Source: CAD feature listing. Evaluate the final solid. Frame: model axes, mm. A direction names the side the tool comes from. Give positions to 0.01 mm unless a question says otherwise; leave off trailing zeros. Loops run counter-clockwise (first coordinate to the right, second up) from the corner with the lowest first, then second, coordinate; pieces in that order, holes last. Notation, with made-up numbers: M 38,-23 L 71,-23 A15 ccw 71,2 Z; hole C 10.5,28 d3. An arc over 180 degrees is marked long. Put each result on its own line as item: value.
from build123d import *

# Parameters (mm, degrees)
F0_W     = 15.4686
F0_H     = 127
F1_DEPTH = 12.7
F2_R     = 2.0193
F3_DEPTH = 6.35
F4_R     = 3.175
F5_DEPTH = 15.875
F6_SIZE  = 1.6002
F8_DEPTH = 25.4


with BuildPart() as f1:
    # F0 (on Right) → F1 (new body)
    with BuildSketch(Plane.YZ):
        Rectangle(F0_W, F0_H)
    extrude(amount=F1_DEPTH)

    # F2 (on Right) → F3 (cut)
    with BuildSketch(Plane.YZ):
        with Locations((0, -55.5625)):
            Circle(F2_R)
    extrude(amount=F3_DEPTH, mode=Mode.SUBTRACT)

    # F4 (on face) → F5 (cut)
    with BuildSketch(Plane(origin=(0, 0, -63.5), x_dir=(1, 0, 0), z_dir=(0, 0, -1))):
        with Locations((6.35, 0)):
            Circle(F4_R)
    extrude(amount=-F5_DEPTH, mode=Mode.SUBTRACT)

    # F6
    f6_edges = [f1.edges().sort_by_distance(p)[0] for p in [
        (6.35, 7.7343, 63.5),
        (6.35, -7.7343, 63.5),
        (0, 0, 63.5),
        (12.7, 0, 63.5),
    ]]
    chamfer(f6_edges, length=F6_SIZE)

    # F7 (on face) → F8 (cut)
    with BuildSketch(Plane(origin=(0, 0, 0), x_dir=(0, -1, 0), z_dir=(-1, 0, 0))):
        Polygon((-3.8227, -43.026294), (-3.8227, -41.502294), (-7.7343, -40.078588), (-7.7343, -44.45), align=None)
        Polygon((-7.7343, 54.206212), (-7.7343, 49.8348), (-3.8227, 51.258506), (-3.8227, 52.782506), align=None)
        Polygon((-7.7343, 48.313412), (-7.7343, 43.942), (-3.8227, 45.365706), (-3.8227, 46.889706), align=None)
        Polygon((-7.7343, 42.420612), (-7.7343, 38.0492), (-3.8227, 39.472906), (-3.8227, 40.996906), align=None)
        Polygon((-7.7343, 36.527812), (-7.7343, 32.1564), (-3.8227, 33.580106), (-3.8227, 35.104106), align=None)
        Polygon((-7.7343, 30.635012), (-7.7343, 26.2636), (-3.8227, 27.687306), (-3.8227, 29.211306), align=None)
        Polygon((-7.7343, 24.742212), (-7.7343, 20.3708), (-3.8227, 21.794506), (-3.8227, 23.318506), align=None)
        Polygon((-7.7343, 18.849412), (-7.7343, 14.478), (-3.8227, 15.901706), (-3.8227, 17.425706), align=None)
        Polygon((-7.7343, 12.956612), (-7.7343, 8.5852), (-3.8227, 10.008906), (-3.8227, 11.532906), align=None)
        Polygon((-7.7343, 7.063812), (-7.7343, 2.6924), (-3.8227, 4.116106), (-3.8227, 5.640106), align=None)
        Polygon((-7.7343, 1.171012), (-7.7343, -3.2004), (-3.8227, -1.776694), (-3.8227, -0.252694), align=None)
        Polygon((-7.7343, -4.721788), (-7.7343, -9.0932), (-3.8227, -7.669494), (-3.8227, -6.145494), align=None)
        Polygon((-7.7343, -10.614588), (-7.7343, -14.986), (-3.8227, -13.562294), (-3.8227, -12.038294), align=None)
        Polygon((-7.7343, -16.507388), (-7.7343, -20.8788), (-3.8227, -19.455094), (-3.8227, -17.931094), align=None)
        Polygon((-7.7343, -22.400188), (-7.7343, -26.7716), (-3.8227, -25.347894), (-3.8227, -23.823894), align=None)
        Polygon((-7.7343, -28.292988), (-7.7343, -32.6644), (-3.8227, -31.240694), (-3.8227, -29.716694), align=None)
        Polygon((-7.7343, -34.185788), (-7.7343, -38.5572), (-3.8227, -37.133494), (-3.8227, -35.609494), align=None)
    extrude(amount=-F8_DEPTH, mode=Mode.SUBTRACT)


solid = f1.part
1. Contact query for a flat-ended pin moving along its axis: P1, Ø0.8, axis at x = 8, z = 22.5, coming from the +Y side. Output: stop coordinate, or through.
Found:
P1: y = 3.82
2. Access query for faces 4 (the flat face through (6, 7.734, -54)), 5 (the flat face through (6.261, 5.806, 9.287)). Directions: +Z, -Z, +X, -X, +Y, -Y. A direction counts if a zero-diameter tool reaches every point of the face in a straight line with its end or side. Return the directions, or none.
Found:
face 4: +Z, -Z, +X, -X, +Y
face 5: +X, -X, +Y
3. Section query A-A (y = 0). Output: boundary loops of the cut face in (x, z) (3 decimals), plus the area to 3 significant figures.
Found:
outline: M 0,-63.5 L 3.175,-63.5 L 3.175,-57.582 L 0,-57.582 Z; M 0,-53.543 L 3.175,-53.543 L 3.175,-47.625 L 9.525,-47.625 L 9.525,-63.5 L 12.7,-63.5 L 12.7,61.9 L 11.1,63.5 L 1.6,63.5 L 0,61.9 Z
area: 1,500 mm^2
4. Draft query along Z for faces 1 (the flat face through (6.261, 5.751, 12.235)), 2 (the flat face through (6, 7.734, 58)), 3 (the flat face through (6.26, 5.81, 15.18)). Return one class per face: pulls with the +Z half, pulls with the -Z half, needs draft (parallel to the pull), parting line crosses it, or undercut.
Found:
face 1: undercut
face 2: needs draft
face 3: undercut
5. Material intervals for line 1 (Z direction, x = 2.55, y = 0); line 2 (Y direction, x = 6.35, z = -57) (3 decimals); line 3 (X direction, y = 0, z = -52.5) (3 decimals), sorted ascending. Write a range as from..to.
Found:
line 1: -63.5..-57.58, -53.54..63.5
line 2: -7.734..-3.175, 3.175..7.734
line 3: 0..3.175, 9.525..12.7
